The listing builds one solid part. Answer for the finished solid, in the listing's coordinates (mm). Round coordinates to 2 decimals unless told otherwise and drop trailing zeros. Write each loop counter-clockwise with the first axis right and the second up, starting at its lowest first coordinate (ties: lowest second). Pieces come first, ordered by that corner, then holes. Notation, with made-up numbers: (-13.75, 19.5) - (2.25, 19.5) arc R18 cw to (2.25, 49.5) - close; hole circle Ø1 at (-31, 20). An arc over 180 degrees is marked (long way). Return JSON: item names as keys, results as strings. Group by question number.
(1) Section B-B, the plane x = 22.3 is taken. Write down the section's boundary in (y, z).
(2) Section A-A, the plane z = 10 is taken. Write down the section's boundary in (x, y), then the cut area to 3 significant figures.
(3) Determine the mould class of faces 1 (the cylindrical face through (36.99, 1.48, -37.15)), 2 (the flat face through (-8, 3, -9)), 3 (the cylindrical face through (37.15, 1.48, 36.99)), 4 (the cylindrical face through (-0.56, 1.48, 12.54)) for opening direction Z: +Z half, -Z half, draft (parallel to the pull), parting line (faces both ways), or undercut.
(4) Section D-D, the plane y = 0.95 is taken. Give the number of separate pieces and of enclosed holes in the cut face, then the cut area to 3 significant figures.
(5) Find the intervals of material crossed by line 1 along X through (y, z) = (2.2, 0); line 2 along Z through (x, y) = (0, 1.6); line 3 along X through (y, z) = (1.9, -22.3), in increasing order. Write a range as [from, to].
(6) Section C-C, the plane x = 10 is taken. Write down the section's boundary in (y, z), then the cut area to 3 significant figures.
```python
from build123d import *

# Parameters (mm, degrees)
SKETCH1_R           = 2.6
SKETCH1_R_2         = 3.55
BOSS_EXTRUDE1_DEPTH = 3


with BuildPart() as part:
    # Sketch1 → Boss-Extrude1 (new body)
    with BuildSketch(Plane(origin=(0, 0, 0), x_dir=(1, 0, 0), z_dir=(0, 1, 0))):
        with BuildLine():
            Line((30, -40), (-30, -40))
            ThreePointArc((-30, -40), (-37.071067812, -37.071067812), (-40, -30))
            Line((-40, -30), (-40, 30))
            ThreePointArc((-40, 30), (-37.071067812, 37.071067812), (-30, 40))
            Line((-30, 40), (30, 40))
            ThreePointArc((30, 40), (37.071067812, 37.071067812), (40, 30))
            Line((40, 30), (40, -30))
            ThreePointArc((40, -30), (37.071067812, -37.071067812), (30, -40))
        make_face()
        Circle(SKETCH1_R, mode=Mode.SUBTRACT)
        with Locations((0, -10)):
            Circle(SKETCH1_R, mode=Mode.SUBTRACT)
        with Locations((-10, 0)):
            Circle(SKETCH1_R, mode=Mode.SUBTRACT)
        with Locations((10, 0)):
            Circle(SKETCH1_R, mode=Mode.SUBTRACT)
        with Locations((0, 10)):
            Circle(SKETCH1_R, mode=Mode.SUBTRACT)
        with Locations((-22.3, 22.3)):
            Circle(SKETCH1_R_2, mode=Mode.SUBTRACT)
        with Locations((-22.3, 0)):
            Circle(SKETCH1_R_2, mode=Mode.SUBTRACT)
        with Locations((-22.3, -22.3)):
            Circle(SKETCH1_R_2, mode=Mode.SUBTRACT)
        with Locations((0, 22.3)):
            Circle(SKETCH1_R, mode=Mode.SUBTRACT)
        with Locations((0, -22.3)):
            Circle(SKETCH1_R, mode=Mode.SUBTRACT)
        with Locations((22.3, 22.3)):
            Circle(SKETCH1_R, mode=Mode.SUBTRACT)
        with Locations((22.3, 0)):
            Circle(SKETCH1_R, mode=Mode.SUBTRACT)
        with Locations((22.3, -22.3)):
            Circle(SKETCH1_R, mode=Mode.SUBTRACT)
    extrude(amount=BOSS_EXTRUDE1_DEPTH)


solid = part.part
```
Working result:
{
 "1": {"outline": "(0, -40) - (3, -40) - (3, -24.9) - (0, -24.9) - close; (0, -19.7) - (3, -19.7) - (3, -2.6) - (0, -2.6) - close; (0, 2.6) - (3, 2.6) - (3, 19.7) - (0, 19.7) - close; (0, 24.9) - (3, 24.9) - (3, 40) - (0, 40) - close"},
 "2": {"outline": "(-40, 0) - (-2.6, 0) - (-2.6, 3) - (-40, 3) - close; (2.6, 0) - (40, 0) - (40, 3) - (2.6, 3) - close", "area": "224 mm^2"},
 "3": {"face 1": "-Z half", "face 2": "draft", "face 3": "+Z half", "face 4": "undercut"},
 "4": {"separate pieces": "1", "enclosed holes": "13", "area": "5,980 mm^2"},
 "5": {"line 1": "x = [-40, -25.85], [-18.75, -12.6], [-7.4, -2.6], [2.6, 7.4], [12.6, 19.7], [24.9, 40]", "line 2": "z = [-40, -24.9], [-19.7, -12.6], [-7.4, -2.6], [2.6, 7.4], [12.6, 19.7], [24.9, 40]", "line 3": "x = [-40, -25.85], [-18.75, -2.6], [2.6, 19.7], [24.9, 40]"},
 "6": {"outline": "(0, -40) - (3, -40) - (3, -2.6) - (0, -2.6) - close; (0, 2.6) - (3, 2.6) - (3, 40) - (0, 40) - close", "area": "224 mm^2"}
}
